```python
from build123d import *

# Parameters (mm, degrees)
SKETCH1_R           = 9
BOSS_EXTRUDE1_DEPTH = 12.5
SKETCH2_R           = 3.175
CUT_EXTRUDE1_DEPTH  = 26
SKETCH3_R           = 1.5
CUT_EXTRUDE2_DEPTH  = 10
SKETCH4_R           = 1.5
CUT_EXTRUDE3_DEPTH  = 10.0000001


with BuildPart() as part:
    # Sketch1 → Boss-Extrude1 (new body, symmetric)
    with BuildSketch(Plane.XY):
        Circle(SKETCH1_R)
    extrude(amount=BOSS_EXTRUDE1_DEPTH, both=True)

    # Sketch2 → Cut-Extrude1 (cut, through all)
    with BuildSketch(Plane.XY.offset(12.5)):
        Circle(SKETCH2_R)
    extrude(amount=-CUT_EXTRUDE1_DEPTH, mode=Mode.SUBTRACT)

    # Sketch3 → Cut-Extrude2 (cut, through all)
    with BuildSketch(Plane(origin=(0, 0, 0), x_dir=(1, 0, 0), z_dir=(0, 1, 0))):
        with Locations((0, 10)):
            Circle(SKETCH3_R)
        with Locations((0, -10)):
            Circle(SKETCH3_R)
    extrude(amount=CUT_EXTRUDE2_DEPTH, mode=Mode.SUBTRACT)

    # Sketch4 → Cut-Extrude3 (cut, through all)
    with BuildSketch(Plane(origin=(0, 0, 0), x_dir=(0, 0, -1), z_dir=(1, 0, 0))):
        with Locations((-10, 0)):
            Circle(SKETCH4_R)
        with Locations((10, 0)):
            Circle(SKETCH4_R)
    extrude(amount=CUT_EXTRUDE3_DEPTH, mode=Mode.SUBTRACT)


solid = part.part
```
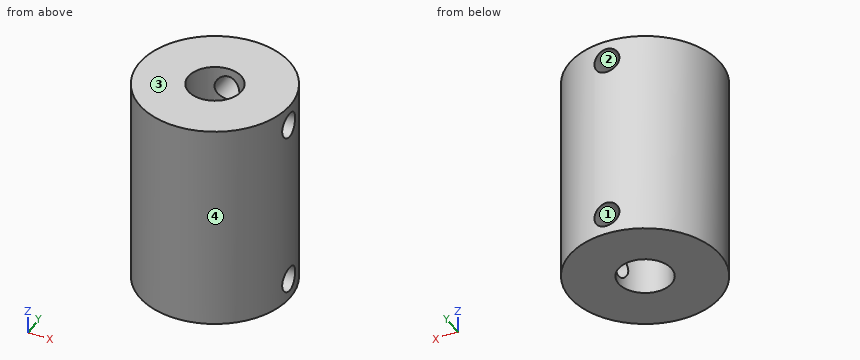
For this review, take the finished solid that the model builds, in its own axes (mm). Face numbers are marked on the shaded views. Round coordinates to 2 decimals unless told otherwise and drop trailing zeros. Write each loop counter-clockwise with the first axis right and the second up, starting at its lowest first coordinate (ties: lowest second). Pieces come first, ordered by that corner, then holes. Notation, with made-up numbers: (81.5, 42) -> (96.5, 42) arc R23 ccw to (96.5, 59) -> close; hole circle Ø4 at (11, -19.75). An arc over 180 degrees is marked (long way). One line per question, with ' | ' between items. Start each with the question number.
1) Add section A-A (y = 0). Write out the cut boundary in (x, z) (3 decimals).
2) Add section C-C (z = -9.5). Write out the cut boundary in (x, y) (3 decimals).
3) Mouldability with a two-part tool opening along X and no side actions: class the marked faces 1, 2, 3 and 4 as +X half, -X half, draft (parallel to the pull), parting line (faces both ways), or undercut.
4) Add section D-D (x = -2). Write out the cut boundary in (y, z), and give its area (3 significant figures).
5) For pin 1 Ø1.8 at (y, z) = (0, 10) entering from +X; pin 2 Ø5 at (y, z) = (-6, -3) entering from +X; pin 3 Ø1 at (y, z) = (2.5, -4) entering from -X, all flat-tipped, find the tip position at first contact; note any pin that passes through.
6) Wall thickness on line 1 along Z through (x, y) = (6.75, 0); line 2 along Y through (x, z) = (0, 3.75) (3 decimals); line 3 along Z through (x, y) = (7.75, -0.5): over which ranges is each line inside the solid? List them lowest first.
Reported:
1) outline: (-9, -12.5) -> (-3.175, -12.5) -> (-3.175, 12.5) -> (-9, 12.5) -> close; (3.175, -12.5) -> (9, -12.5) -> (9, -11.5) -> (3.175, -11.5) -> close; (3.175, -8.5) -> (9, -8.5) -> (9, 8.5) -> (3.175, 8.5) -> close; (3.175, 11.5) -> (9, 11.5) -> (9, 12.5) -> (3.175, 12.5) -> close
2) outline: (-1.414, 2.843) -> (-1.414, 8.888) arc R9 ccw (long way) to (8.888, -1.414) -> (2.843, -1.414) arc R3.175 cw (long way) to start; (1.414, 2.843) arc R3.175 cw to (2.843, 1.414) -> (8.888, 1.414) arc R9 ccw to (1.414, 8.888) -> close
3) face 1: undercut | face 2: undercut | face 3: draft | face 4: parting line
4) outline: (-8.77, -12.5) -> (-2.47, -12.5) -> (-2.47, 12.5) -> (-8.77, 12.5) -> close; (2.47, -12.5) -> (8.77, -12.5) -> (8.77, 12.5) -> (2.47, 12.5) -> close | area: 315 mm²
5) pin 1: stops at x = -3.04 | pin 2: stops at x = 8.29 | pin 3: stops at x = -8.77
6) line 1: z = -12.5 to -11.5, -8.5 to 8.5, 11.5 to 12.5 | line 2: y = -9 to -3.175, 3.175 to 9 | line 3: z = -12.5 to -11.41, -8.59 to 8.59, 11.41 to 12.5
